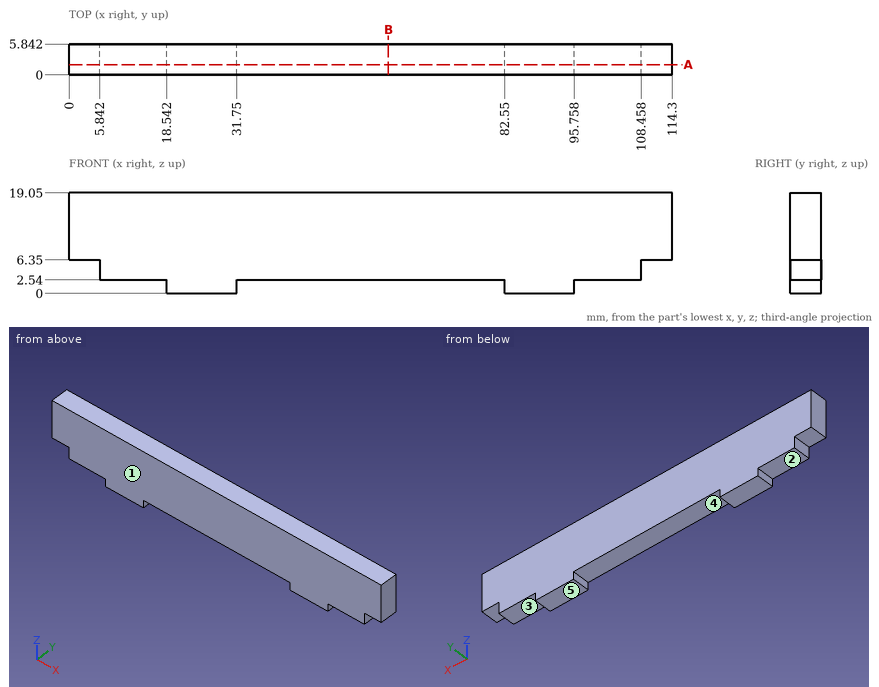
Could you check a few things on this drawing? It's one solid part, dimensions in mm from its lowest x, y, z. A direction names the side the tool comes from. Coordinates: 2 decimals unless noted, no trailing zeros. Write each loop counter-clockwise with the first axis right and the second up, starting at its lowest first coordinate (ties: lowest second). Pieces come first, ordered by that corner, then holes. Notation, with made-up numbers: (-31.75, 59.5) - (-20.75, 59.5) arc R20 ccw to (-20.75, 86.5) - close; hole circle Ø3 at (33, 15). An arc over 180 degrees is marked (long way). Return JSON: item names as keys, results as strings. Group by question number.
Item 1: Which directions (+Z, -Z, +X, -X, +Y, -Y) give clear straight access to the entire face, cutting with the end or side of a thin tool? Please do the marked faces 1, 2 and 3.
Item 2: We'd pull the mould along X, two halves only. Please class the marked faces 4 and 5: pulls with the +X half, pulls with the -X half, needs draft (parallel to the pull), parting line crosses it, or undercut.
Item 3: I'm going to push flat-ended pins straight in: pin 1 Ø3 at (x, y) = (111.5, 3.5) entering from -Z; pin 2 Ø1.1 at (y, z) = (2, 4.5) entering from -X; pin 3 Ø1.1 at (y, z) = (2.5, 5) entering from +X. Where does each tip first touch, or does it pass through?
Item 4: If we section it at B-B (x = 60.5): Write out the boundary of the cut face in (y, z).
Item 5: If we section it at A-A (y = 1.95): Write out the boundary of the cut face in (x, z), then the cut area to 3 significant figures.
Item 6: Please list where these lines run through material, in increasing order: probe 1 along Z at (x, y) = (46.5, 0.5); probe 2 along X at (y, z) = (4.7, 1).
Return value:
{
 "1": {"face 1": "+Z, -Z, +X, -X, -Y", "face 2": "-Z, -X, +Y, -Y", "face 3": "-Z, +X, +Y, -Y"},
 "2": {"face 4": "undercut", "face 5": "needs draft"},
 "3": {"pin 1": "stops at z = 6.35", "pin 2": "stops at x = 5.84", "pin 3": "stops at x = 108.46"},
 "4": {"outline": "(0, 2.54) - (5.84, 2.54) - (5.84, 19.05) - (0, 19.05) - close"},
 "5": {"outline": "(0, 6.35) - (5.84, 6.35) - (5.84, 2.54) - (18.54, 2.54) - (18.54, 0) - (31.75, 0) - (31.75, 2.54) - (82.55, 2.54) - (82.55, 0) - (95.76, 0) - (95.76, 2.54) - (108.46, 2.54) - (108.46, 6.35) - (114.3, 6.35) - (114.3, 19.05) - (0, 19.05) - close", "area": "1,910 mm^2"},
 "6": {"probe 1": "z = 2.54 to 19.05", "probe 2": "x = 18.54 to 31.75, 82.55 to 95.76"}
}
